Geometry check sheet. Reference: the model listing, model coordinates, mm. A direction names the side the tool comes from. Round coordinates to 2 decimals unless told otherwise and drop trailing zeros. Order: outer loops, then holes, each group sorted by start corner. A loop starts at its lowest first (then second) coordinate and runs counter-clockwise, first axis right, second up. Notation, with made-up numbers: (33.25, 25.5) -> (78.25, 25.5) arc R14 ccw to (78.25, 49.5) -> close; hole circle Ø6 at (89.5, 6). An arc over 180 degrees is marked (long way). Answer as a JSON object with one key per item and string values. Group by question number.
from build123d import *

# Parameters (mm, degrees)
EXTRUIR1_DEPTH      = 20
EXTRUIR2_REACH      = 80.184
EXTRUIR2_END_RADIUS = 23
EXTRUIR2_START      = 40
CROQUIS2_R          = 4
REDONDEO1_R         = 3
REDONDEO2_R         = 0.5


with BuildPart() as part:
    # Croquis1 → Extruir1 (new body)
    with BuildSketch(Plane(origin=(0, 0, 0), x_dir=(1, 0, 0), z_dir=(0, 1, 0))):
        with BuildLine():
            Line((19.918584287, 11.5), (17.320508076, 10))
            ThreePointArc((17.320508076, 10), (0, -20), (-17.320508076, 10))
            Line((-17.320508076, 10), (-19.918584287, 11.5))
            ThreePointArc((-19.918584287, 11.5), (0, -23), (19.918584287, 11.5))
        make_face()
    extrude(amount=EXTRUIR1_DEPTH)

    # Extruir2: up to this cylinder (the profile starts outside it)
    extruir2_end = Plane(origin=(0, 10, 0), z_dir=(0, -1, 0)) * Cylinder(EXTRUIR2_END_RADIUS, 207.368, mode=Mode.PRIVATE)
    # Croquis2 → Extruir2 (add, up to the surface)
    with BuildSketch(Plane.XY.offset(EXTRUIR2_START), mode=Mode.PRIVATE) as extruir2_sk1:
        with Locations((0, 10)):
            Circle(CROQUIS2_R)
    extruir2_tool1 = extrude(extruir2_sk1.sketch, amount=-EXTRUIR2_REACH, mode=Mode.PRIVATE) - extruir2_end
    add(extruir2_tool1.solids().sort_by_distance((0, 10, 40))[0])

    # Redondeo1
    redondeo1_edges = [part.edges().sort_by_distance(p)[0] for p in [
        (17.320508076, 10, -10),
        (-17.320508076, 10, -10),
    ]]
    fillet(redondeo1_edges, radius=REDONDEO1_R)

    # Redondeo2
    redondeo2_edges = [part.edges().sort_by_distance(p)[0] for p in [
        (19.918584287, 10, -11.5),
        (-19.918584287, 10, -11.5),
    ]]
    fillet(redondeo2_edges, radius=REDONDEO2_R)


solid = part.part
Item 1: Sectioned sample at B-B, the plane x = 0. Enter the section's corners in (y, z), then the cut area to 3 significant figures.
Item 2: Set-up check for faces 1 (the flat face through (0, 10, 40)), 2 (the cylindrical face through (-0.521, 13.966, 31.446)), 3 (the cylindrical face through (-18.346, 10.14, -9.563)): record each of +Z, -Z, +X, -X, +Y, -Y from which the full face is reachable in a straight line by a thin tool's end or side.
Item 3: Sectioned sample at A-A, the plane z = 0. Enter the section's corners in (x, y), then the cut area to 3 significant figures.
Item 4: Thickness scan on L1, parallel to X at y = 5.75, z = 0; L2, parallel to X at y = 8.75, z = 17; L3, parallel to Z at x = 0, y = 6.5. Record the ranges inside material, lowest first.
Item 5: Depth check by flat-ended pin: pin 1 Ø3 at (y, z) = (11.5, 17.5) entering from -X; pin 2 Ø12 at (x, y) = (16, 4) entering from +Z; pin 3 Ø4 at (x, y) = (-15, 6.5) entering from +Z. Enter the tip coordinate at first touch or a pass-through.
Item 6: Sectioned sample at C-C, the plane z = 6. Enter the section's corners in (x, y), then the cut area to 3 significant figures.
Item 7: Mould release check, pull along X, two halves, no side actions. Record for faces 4 (the cylindrical face through (0.55, 9.86, 19.992)), 5 (the cylindrical face through (-0.67, 5.42, 22.99)), 6 (the flat face through (-4, 0, 20)): pulls with the +X half, pulls with the -X half, needs draft (parallel to the pull), parting line crosses it, or undercut.
Item 8: Sectioned sample at D-D, the plane z = 31. Enter the section's corners in (x, y), then the cut area to 3 significant figures.
Result:
{
 "1": {"outline": "(0, 20) -> (20, 20) -> (20, 23) -> (14, 23) -> (14, 40) -> (6, 40) -> (6, 23) -> (0, 23) -> close", "area": "196 mm2"},
 "2": {"face 1": "+Z, +X, -X, +Y, -Y", "face 2": "+Z", "face 3": "+Y, -Y"},
 "3": {"outline": "(-23, 0) -> (-20, 0) -> (-20, 20) -> (-23, 20) -> close; (20, 0) -> (23, 0) -> (23, 20) -> (20, 20) -> close", "area": "120 mm2"},
 "4": {"L1": "x = -23 to -20, 20 to 23", "L2": "x = -15.49 to -10.54, 10.54 to 15.49", "L3": "z = 20 to 40"},
 "5": {"pin 1": "stops at x = -16.52", "pin 2": "stops at z = 20.71", "pin 3": "stops at z = 18.97"},
 "6": {"outline": "(-22.2, 0) -> (-19.08, 0) -> (-19.08, 20) -> (-22.2, 20) -> close; (19.08, 0) -> (22.2, 0) -> (22.2, 20) -> (19.08, 20) -> close", "area": "125 mm2"},
 "7": {"face 4": "undercut", "face 5": "parting line crosses it", "face 6": "needs draft"},
 "8": {"outline": "circle Ø8 at (0, 10)", "area": "50.3 mm2"}
}
